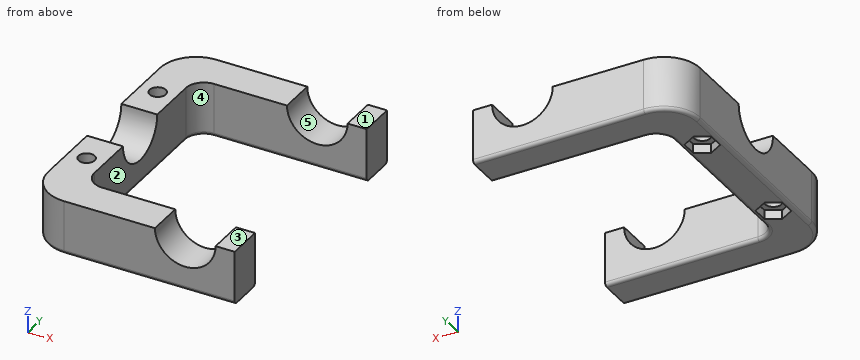
from build123d import *

# Parameters (mm, degrees)
F0_W      = 60
F0_H      = 60
F0_W_2    = 44
F0_H_2    = 44
F1_DEPTH  = 12
F3_DEPTH  = 25
F4_R      = 8
F5_R      = 4
F7_DEPTH  = 25
F9_DEPTH  = 60.001
F10_R     = 1.8
F11_DEPTH = 25
F12_R     = 0.8
F13_R     = 1.8
F14_DEPTH = 2


# Not quite as in the source:
# - a feature names something its author has since deleted; it is built from what else it names


with BuildPart() as f1:
    # F0 (on Top) → F1 (new body)
    with BuildSketch(Plane.XY):
        Rectangle(F0_W, F0_H)
        Rectangle(F0_W_2, F0_H_2, mode=Mode.SUBTRACT)
    extrude(amount=F1_DEPTH)

    # F2 (on face) → F3 (cut)
    with BuildSketch(Plane.XY.offset(12)):
        Polygon((30, -30), (30, 30), (16, 30), (16, 22), (22, 22), (22, -22), (16, -22), (16, -30), align=None)
    extrude(amount=-F3_DEPTH, mode=Mode.SUBTRACT)

    # F4
    f4_edges = [f1.edges().sort_by_distance(p)[0] for p in [
        (-30, -30, 6),
        (-30, 30, 6),
    ]]
    fillet(f4_edges, radius=F4_R)

    # F5
    f5_edges = [f1.edges().sort_by_distance(p)[0] for p in [
        (-22, 22, 6),
        (-22, -22, 6),
    ]]
    fillet(f5_edges, radius=F5_R)

    # F6 (on face) → F7 (cut)
    with BuildSketch(Plane.YZ.offset(-22)):
        with BuildLine():
            ThreePointArc((-6.75, 12), (0, 5.25), (6.75, 12))
            Line((6.75, 12), (-6.75, 12))
        make_face()
    extrude(amount=-F7_DEPTH, mode=Mode.SUBTRACT)

    # F8 (on face) → F9 (cut, through all)
    with BuildSketch(Plane.XZ.offset(30)):
        with BuildLine():
            ThreePointArc((-1.75, 12), (5, 5.25), (11.75, 12))
            Line((11.75, 12), (-1.75, 12))
        make_face()
    extrude(amount=-F9_DEPTH, mode=Mode.SUBTRACT)

    # F10 (on face) → F11 (cut)
    with BuildSketch(Plane.XY.offset(12)):
        with Locations((-26, 14)):
            Circle(F10_R)
        with Locations((-26, -14)):
            Circle(F10_R)
    extrude(amount=-F11_DEPTH, mode=Mode.SUBTRACT)

    # F12
    f12_edges = [f1.edges().sort_by_distance(p)[0] for p in [
        (-3, -30, 0),
        (-20.828427, 20.828427, 0),
    ]]
    fillet(f12_edges, radius=F12_R)

    # F13 (on face) → F14 (cut)
    with BuildSketch(Plane(origin=(0, 0, 0), x_dir=(1, 0, 0), z_dir=(0, 0, -1))):
        Polygon((-23, 12.2679491924), (-23, 15.7320508076), (-26, 17.4641016151), (-29, 15.7320508076), (-29, 12.2679491924), (-26, 10.5358983849), align=None)
        with Locations((-26, 14)):
            Circle(F13_R, mode=Mode.SUBTRACT)
        Polygon((-26, -17.4641016151), (-23, -15.7320508076), (-23, -12.2679491924), (-26, -10.5358983849), (-29, -12.2679491924), (-29, -15.7320508076), align=None)
        with Locations((-26, -14)):
            Circle(F13_R, mode=Mode.SUBTRACT)
    extrude(amount=-F14_DEPTH, mode=Mode.SUBTRACT)


solid = f1.part
Geometry check sheet. Reference: the model listing, model coordinates, mm. Face numbers are marked on the shaded views. A direction names the side the tool comes from. Round coordinates to 2 decimals unless told otherwise and drop trailing zeros. Order: outer loops, then holes, each group sorted by start corner. A loop starts at its lowest first (then second) coordinate and runs counter-clockwise, first axis right, second up. Notation, with made-up numbers: M -25,27 L 15,27 A23 ccw 15,53 Z; hole C 66.5,-36.5 d1. An arc over 180 degrees is marked long. Answer in a Markdown table with one row per item. Add a question column.
Item 1: Sectioned sample at B-B, the plane x = 5. Enter the section's corners in (y, z), plus the area to 3 significant figures.
Item 2: Set-up check for the marked faces 1 and 2: record each of +Z, -Z, +X, -X, +Y, -Y from which the full face is reachable in a straight line by a thin tool's end or side.
Item 3: Material ranges on L1, parallel to Y at x = -17.5, z = 10; L2, parallel to Y at x = -26, z = 9.25; L3, parallel to X at y = 14, z = 6.75, recorded low to high. Write a range as [from, to].
Item 4: Depth check by flat-ended pin: pin 1 Ø4.5 at (x, y) = (-26, -14) entering from +Z; pin 2 Ø2 at (y, z) = (14.5, 0.5) entering from +X; pin 3 Ø5 at (x, y) = (7, 24) entering from +Z. Enter the tip coordinate at first touch or a pass-through.
Item 5: Sectioned sample at C-C, the plane z = 11. Enter the section's corners in (x, y).
Item 6: Sectioned sample at A-A, the plane y = -14. Enter the section's corners in (x, z).
Item 7: Draft check along X on the marked faces 3, 4 and 5. Enter one of: released by +X, released by -X, zero draft, split by the parting line, or undercut.
Item 8: Sectioned sample at D-D, the plane z = 7.75. Enter the section's corners in (x, y), plus the area to 3 significant figures.
Filled in:
| question | item | result |
|---|---|---|
| 1 | outline | M -30,0.8 A0.8 ccw -29.2,0 L -22.8,0 A0.8 ccw -22,0.8 L -22,5.25 L -30,5.25 Z; M 22,0.8 A0.8 ccw 22.8,0 L 29.2,0 A0.8 ccw 30,0.8 L 30,5.25 L 22,5.25 Z |
| 1 | area | 83.5 mm² |
| 2 | face 1 | +Z, +X, -X, +Y, -Y |
| 2 | face 2 | +Z, -Z, +X |
| 3 | L1 | y = [-30, -22], [22, 30] |
| 3 | L2 | y = [-28.93, -15.8], [-12.2, -6.16], [6.16, 12.2], [15.8, 28.93] |
| 3 | L3 | x = [-30, -27.8], [-24.2, -22] |
| 4 | pin 1 | stops at z = 12 |
| 4 | pin 2 | stops at x = -22 |
| 4 | pin 3 | stops at z = 6.97 |
| 5 | outline | M -30,-22 A8 ccw -22,-30 L -1.68,-30 L -1.68,-22 L -18,-22 A4 cw -22,-18 L -22,-6.68 L -30,-6.68 Z; M -30,6.68 L -22,6.68 L -22,18 A4 cw -18,22 L -1.68,22 L -1.68,30 L -22,30 A8 ccw -30,22 Z; M 11.68,-30 L 16,-30 L 16,-22 L 11.68,-22 Z; M 11.68,22 L 16,22 L 16,30 L 11.68,30 Z; hole C -26,-14 d3.6; hole C -26,14 d3.6 |
| 6 | outline | M -30,0.8 A0.8 ccw -29.2,0 L -29,0 L -29,2 L -27.8,2 L -27.8,12 L -30,12 Z; M -24.2,2 L -23,2 L -23,0 L -22.8,0 A0.8 ccw -22,0.8 L -22,12 L -24.2,12 Z |
| 7 | face 3 | zero draft |
| 7 | face 4 | released by +X |
| 7 | face 5 | undercut |
| 8 | outline | M -30,-22 A8 ccw -22,-30 L -0.24,-30 L -0.24,-22 L -18,-22 A4 cw -22,-18 L -22,-5.24 L -30,-5.24 Z; M -30,5.24 L -22,5.24 L -22,18 A4 cw -18,22 L -0.24,22 L -0.24,30 L -22,30 A8 ccw -30,22 Z; M 10.24,-30 L 16,-30 L 16,-22 L 10.24,-22 Z; M 10.24,22 L 16,22 L 16,30 L 10.24,30 Z; hole C -26,-14 d3.6; hole C -26,14 d3.6 |
| 8 | area | 795 mm² |
